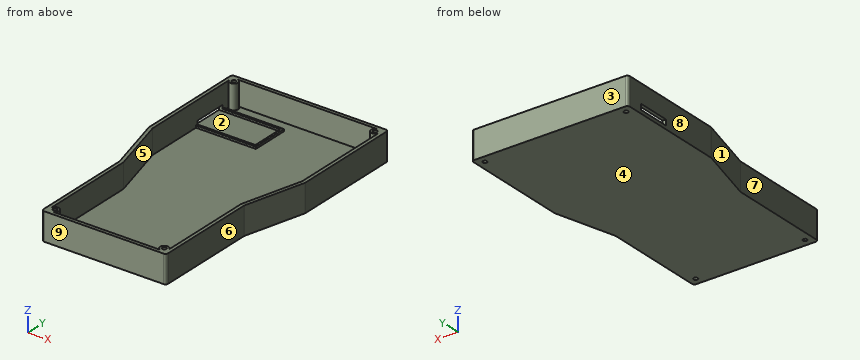
from build123d import *

# Parameters (mm, degrees)
BOSS_EXTRUDE1_DEPTH = 20
SHELL1_T            = -2.5
FILLET1_R           = 2
BOSS_EXTRUDE2_DEPTH = 17.5
SKETCH4_R           = 1.5
CUT_EXTRUDE1_DEPTH  = 208.327218727
BOSS_EXTRUDE3_DEPTH = 1.5
CUT_EXTRUDE2_REACH  = 231.263
SKETCH6_W           = 4
SKETCH6_H           = 24


with BuildPart() as part:
    # Sketch1 → Boss-Extrude1 (new body)
    with BuildSketch(Plane.XY):
        Polygon((-45, -123.475), (-45, -198.475), (45, -198.475), (45, -123.475), (56.5, -79.95), (56.5, 0), (-56.5, 0), (-56.5, -79.95), align=None)
    extrude(amount=BOSS_EXTRUDE1_DEPTH)

    # Shell1
    shell1_openings = [part.faces().sort_by_distance(p)[0] for p in [
        (0, -93.724865495, 20),
    ]]
    offset(amount=SHELL1_T, openings=shell1_openings, kind=Kind.INTERSECTION)

    # Fillet1
    fillet1_edges = [part.edges().sort_by_distance(p)[0] for p in [
        (-56.5, -79.95, 10),
        (-56.5, 0, 10),
        (56.5, 0, 10),
        (56.5, -79.95, 10),
        (45, -123.475, 10),
        (45, -198.475, 10),
        (-45, -198.475, 10),
        (-45, -123.475, 10),
    ]]
    fillet(fillet1_edges, radius=FILLET1_R)

    # Sketch2 → Boss-Extrude2 (add, through all)
    with BuildSketch(Plane.XY.offset(2.5)):
        with BuildLine():
            Line((54, -5.5), (54, -2.5))
            Line((54, -2.5), (51, -2.5))
            ThreePointArc((51, -2.5), (48.878679656, -7.621320344), (54, -5.5))
        make_face()
        with BuildLine():
            Line((42.5, -195.975), (42.5, -192.975))
            ThreePointArc((42.5, -192.975), (37.378679656, -190.853679656), (39.5, -195.975))
            Line((39.5, -195.975), (42.5, -195.975))
        make_face()
        with BuildLine():
            Line((-39.5, -195.975), (-42.5, -195.975))
            Line((-42.5, -195.975), (-42.5, -192.975))
            ThreePointArc((-42.5, -192.975), (-37.378679656, -190.853679656), (-39.5, -195.975))
        make_face()
        with BuildLine():
            Line((-54, -2.5), (-51, -2.5))
            ThreePointArc((-51, -2.5), (-48.878679656, -7.621320344), (-54, -5.5))
            Line((-54, -5.5), (-54, -2.5))
        make_face()
    extrude(amount=BOSS_EXTRUDE2_DEPTH)

    # Sketch4 → Cut-Extrude1 (cut, through all)
    with BuildSketch(Plane.XY.offset(20)):
        with Locations((51, -5.5)):
            Circle(SKETCH4_R)
        with Locations((39.5, -192.975)):
            Circle(SKETCH4_R)
        with Locations(Location((-39.5, -192.975, 0), (0, 0, 180))):
            Circle(SKETCH4_R)
        with Locations(Location((-51, -5.5, 0), (0, 0, 180))):
            Circle(SKETCH4_R)
    extrude(amount=-CUT_EXTRUDE1_DEPTH, mode=Mode.SUBTRACT)

    # Sketch5 → Boss-Extrude3 (add)
    with BuildSketch(Plane.XY.offset(2.5)):
        Polygon((-54, -11), (-54, -12.5), (-12.2, -12.5), (-12.2, -36.5), (-54, -36.5), (-54, -38), (-10.7, -38), (-10.7, -11), align=None)
    extrude(amount=BOSS_EXTRUDE3_DEPTH)

    # Sketch6 → Cut-Extrude2 (cut, up to next)
    with BuildSketch(Plane.ZY.offset(56.5), mode=Mode.PRIVATE) as cut_extrude2_sk1:
        with Locations((4.5, -24.5)):
            Rectangle(SKETCH6_W, SKETCH6_H)
    cut_extrude2_tool1 = extrude(cut_extrude2_sk1.sketch, amount=-CUT_EXTRUDE2_REACH, mode=Mode.PRIVATE) & part.part
    add(cut_extrude2_tool1.solids().sort_by_distance((-56.5, -24.5, 4.5))[0], mode=Mode.SUBTRACT)


solid = part.part
Build history of the part. All positions in model axes, mm. Face numbers are marked on the shaded views. A direction names the side the tool comes from. Round coordinates to 2 decimals unless told otherwise and drop trailing zeros. Write each loop counter-clockwise with the first axis right and the second up, starting at its lowest first coordinate (ties: lowest second). Pieces come first, ordered by that corner, then holes. Notation, with made-up numbers: (-24, 54.25) -> (23, 54.25) arc R16 cw to (23, 77.25) -> close; hole circle Ø4 at (74, -8.75). An arc over 180 degrees is marked (long way). Write item = value, one per line.
(1) Band-saw the part on D-D (x = -20). Give the cut face in (y, z) (3 decimals).
Answer:
outline = (-198.475, 0) -> (0, 0) -> (0, 20) -> (-2.5, 20) -> (-2.5, 2.5) -> (-11, 2.5) -> (-11, 4) -> (-12.5, 4) -> (-12.5, 2.5) -> (-36.5, 2.5) -> (-36.5, 4) -> (-38, 4) -> (-38, 2.5) -> (-195.975, 2.5) -> (-195.975, 20) -> (-198.475, 20) -> close
(2) Flat gauge pins, fed straight in: pin 1 (2 mm diameter, centred on y = -85.5, z = 5.5, fed in from -X); pin 2 (13.5 mm diameter, centred on x = -22, y = -19.5, fed in from +Z); pin 3 (8 mm diameter, centred on x = -16, y = -116, fed in from -Z); pin 4 (5 mm diameter, centred on y = -171.5, z = 7, fed in from -X). Where does each tip first touch, or does it go through?
Answer:
pin_1 = -55.3
pin_2 = 2.5
pin_3 = 0
pin_4 = -45
(3) Tool access for the marked faces 5, 6, 7, 8 and 9: list every direction of +Z, -Z, +X, -X, +Y, -Y with a clear straight run to the whole face (end or side of a thin tool).
Answer:
face_5 = +Z
face_6 = +Z, -Z, +X, -Y
face_7 = +Z, -Z, -X, -Y
face_8 = +Z, -Z, -X, +Y, -Y
face_9 = +Z, -Z, +X, -X, -Y
(4) Probe L1, parallel to Y at x = -13.5, z = 3 (3 decimals); L2, parallel to Y at x = -7.5, z = 7.25 (3 decimals); L3, parallel to X at y = -124, z = 5.75. List the from-to ranges inside material, lowest first.
Answer:
L1 = -198.475 to -195.975, -38 to -36.5, -12.5 to -11, -2.5 to 0
L2 = -198.475 to -195.975, -2.5 to 0
L3 = -45 to -42.5, 42.5 to 45
(5) Band-saw the part on B-B (y = -69). Give the cut face in (x, z), then the cut area to 3 significant figures.
Answer:
outline = (-56.5, 0) -> (56.5, 0) -> (56.5, 20) -> (54, 20) -> (54, 2.5) -> (-54, 2.5) -> (-54, 20) -> (-56.5, 20) -> close
area = 370 mm2
(6) Band-saw the part on C-C (z = 9). State how many separate pieces and enclosed holes the cut face has, then the cut area to 3 significant figures.
Answer:
separate_pieces = 1
enclosed_holes = 5
area = 1,570 mm2
(7) Band-saw the part on A-A (x = 29). Give the cut face in (y, z) (3 decimals).
Answer:
outline = (-198.475, 0) -> (0, 0) -> (0, 20) -> (-2.5, 20) -> (-2.5, 2.5) -> (-195.975, 2.5) -> (-195.975, 20) -> (-198.475, 20) -> close
(8) Two-plate mould, pull along Y, no slides. Class the marked faces 1, 2, 3 and 4: pulls with the +Y half, pulls with the -Y half, needs draft (parallel to the pull), parting line crosses it, or undercut.
Answer:
face_1 = pulls with the -Y half
face_2 = undercut
face_3 = pulls with the +Y half
face_4 = needs draft
